Autodesk Inventor part; units mm, degrees
ref_plane "Work Plane1" through (-2.1808, -2.1808, 614.9086) normal (-0.7071068, 0.7071068, 0) x (0, 0, 1)
ref_plane "YZ Plane" through (0, 0, 0) normal (1, 0, 0) x (0, 1, 0)
ref_plane "XZ Plane" through (0, 0, 0) normal (0, 1, 0) x (-1, 0, 0)
sketch "Sketch1" plane through (0, 0, 0) normal (0, 0, 1) x (1, 0, 0)
  line L0 (-5.3558, -5.3558) -> (5.3558, -5.3558)
  line L1 (5.3558, -5.3558) -> (5.3558, 5.3558)
  line L2 (5.3558, 5.3558) -> (-5.3558, 5.3558)
  line L3 (-5.3558, 5.3558) -> (-5.3558, -5.3558)
  line L4 (-5.3558, -5.3558) -> (5.3558, 5.3558) construction
  line L5 (5.3558, -5.3558) -> (-5.3558, 5.3558) construction
  line L6 (5.3558, 5.3558) -> (-2.1808, 5.3558)
  line L7 (-2.1808, 5.3558) -> (-2.1808, -2.1808)
  line L8 (-2.1808, -2.1808) -> (5.3558, -2.1808)
  line L9 (5.3558, -2.1808) -> (5.3558, 5.3558)
  point P0 (0, 0)
  dimension "d0" = 3.175
  dimension "d1" = 3.175
extrude "Extrusion1" add sketch "Sketch1" along normal blind 618.0836 contours L3 L2 L7 L8 L1 L0
sketch "Sketch2" plane through (-5.3558, -5.3558, 0) normal (-1, 0, 0) x (0, 0, 1)
  line L0 (0, 10.7115) -> (0, 0)
  line L1 (0, 0) -> (618.0836, 0)
  line L2 (0, 10.7115) -> (618.0836, 10.7115)
  line L3 (309.0418, 10.7115) -> (309.0418, 0)
  line L4 (618.0836, 0) -> (607.3721, 10.7115)
  line L5 (618.0836, 0) -> (633.232, 0) construction
  line L6 (607.3721, 10.7115) -> (618.0836, 10.7115)
  line L7 (618.0836, 0) -> (618.0836, 10.7115)
  line L8 (0, 10.7115) -> (0, 0)
  line L9 (0, 0) -> (10.7115, 10.7115)
  line L10 (0, 0) -> (-15.1484, 0) construction
  line L11 (10.7115, 10.7115) -> (0, 10.7115)
  line L12 (0, 0) -> (0, 10.7115)
  point P0 (0, 5.3558)
  dimension "d4" = 135
extrude "Extrusion2" cut sketch "Sketch2" against normal blind 25.4 contours L2 L9 L0 | L4 L2 L7
ref_plane "Work Plane1" through (-2.1808, -2.1808, 614.9086) normal (-0.7071068, 0.7071068, 0) x (0, 0, 1)
mirror "Mirror1" about plane through (-2.1808, -2.1808, 614.9086) normal (-0.7071068, 0.7071068, 0) of "Extrusion2"
properties part number "2222_Brass Angle Bracket_V1" material "Brass"
Build history of the part. All positions in model axes, mm. Round coordinates to 2 decimals unless told otherwise and drop trailing zeros. Write each loop counter-clockwise with the first axis right and the second up, starting at its lowest first coordinate (ties: lowest second). Pieces come first, ordered by that corner, then holes. Notation, with made-up numbers: M 26.5,77.25 L 67.5,77.25 A27 cw 67.5,114.25 Z; hole C 46.25,71.5 d9. An arc over 180 degrees is marked long. Answer as a JSON object with one key per item and string values. Group by question number.
(1) Cut at A-A (z = 306.5). Give the cut face in (x, y), and give its area (3 significant figures).
(2) Drill centre lines: L1, parallel to Y at x = 2.75, z = 211; L2, parallel to Z at x = -3.5, y = 2. Where is each one in solid material? Low to high.
(3) Cut at C-C (x = 2.25). Give the cut face in (y, z).
(4) Flat gauge pins, fed straight in: pin 1 (6 mm diameter, centred on x = 4, z = 455.5, fed in from +Y); pin 2 (2 mm diameter, centred on x = -3.5, y = -2, fed in from -Z); pin 3 (1 mm diameter, centred on y = 4.5, z = 64.5, fed in from +X). Where does each tip first touch, or does it go through?
(5) Cut at B-B (y = -0.5). Give the cut face in (x, z).
Responses:
{
 "1": {"outline": "M -5.36,-5.36 L 5.36,-5.36 L 5.36,-2.18 L -2.18,-2.18 L -2.18,5.36 L -5.36,5.36 Z", "area": "57.9 mm2"},
 "2": {"L1": "y = -5.36 to -2.18", "L2": "z = 7.36 to 610.73"},
 "3": {"outline": "M -5.36,7.61 L -2.18,7.61 L -2.18,610.48 L -5.36,610.48 Z"},
 "4": {"pin 1": "stops at y = -2.18", "pin 2": "stops at z = 2.36", "pin 3": "stops at x = -2.18"},
 "5": {"outline": "M -5.36,4.86 L -2.18,4.86 L -2.18,613.23 L -5.36,613.23 Z"}
}
